from build123d import *

# Parameters (mm, degrees)
BOSS_EXTRUDE2_DEPTH      = 2
BOSS_EXTRUDE2_DEPTH_BACK = 2
SKETCH1_3_W              = 45
SKETCH1_3_H              = 20
BOSS_EXTRUDE3_DEPTH      = 35
M3_5_CLEARANCE_HOLE2_D   = 3.9
M6_CLEARANCE_HOLE2_D     = 6.6


with BuildPart() as part:
    # Sketch1<3> → Boss-Extrude2 (new, two sides: drawn at the far end of the back side and taken through both)
    with BuildSketch(Plane.XY.offset(-BOSS_EXTRUDE2_DEPTH_BACK)):
        with BuildLine():
            Line((-18.78, 17.478483309), (-8.78, 17.478483309))
            Line((-8.78, 17.478483309), (-8.78, 27.45))
            ThreePointArc((-8.78, 27.45), (-13.78, 32.45), (-18.78, 27.45))
            Line((-18.78, 27.45), (-18.78, 17.478483309))
        make_face()
        Polygon((-18.78, -10), (-18.78, -17.478483309), (-8.78, -17.478483309), (-8.78, 17.478483309), (-18.78, 17.478483309), (-18.78, 10), align=None)
        with BuildLine():
            Line((-8.78, -17.478483309), (-18.78, -17.478483309))
            Line((-18.78, -17.478483309), (-18.78, -27.45))
            ThreePointArc((-18.78, -27.45), (-13.78, -32.45), (-8.78, -27.45))
            Line((-8.78, -27.45), (-8.78, -17.478483309))
        make_face()
        with Locations((-41.28, 0)):
            Rectangle(SKETCH1_3_W, SKETCH1_3_H)
        Polygon((-63.78, -25), (-63.78, -10), (-63.78, 10), (-63.78, 25), (-66.78, 25), (-66.78, -25), align=None)
    extrude(amount=BOSS_EXTRUDE2_DEPTH + BOSS_EXTRUDE2_DEPTH_BACK)

    # Sketch1<4> → Boss-Extrude3 (add)
    with BuildSketch(Plane.XY):
        Polygon((-63.78, -25), (-63.78, -10), (-63.78, 10), (-63.78, 25), (-66.78, 25), (-66.78, -25), align=None)
    extrude(amount=BOSS_EXTRUDE3_DEPTH)

    # M3.5 Clearance Hole2 (through all)
    with Locations(Plane(origin=(0, 0, -2), x_dir=(-1, 0, 0), z_dir=(0, 0, -1))):
        with Locations((13.78, 27.45), (13.78, -27.45)):
            Hole(M3_5_CLEARANCE_HOLE2_D / 2)

    # M6 Clearance Hole2 (through all)
    with Locations(Plane(origin=(-63.78, 0, 0), x_dir=(0, 0, -1), z_dir=(1, 0, 0))):
        with Locations((-29, 19)):
            m6_clearance_hole2 = Hole(M6_CLEARANCE_HOLE2_D / 2)

    # Mirror1: M6 Clearance Hole2 across plane
    add(m6_clearance_hole2.mirror(Plane.ZX), mode=Mode.SUBTRACT)


solid = part.part
CAD build for the part. Positions are in the model's coordinates, mm. A direction names the side the tool comes from. Round coordinates to 2 decimals unless told otherwise and drop trailing zeros. Write each loop counter-clockwise with the first axis right and the second up, starting at its lowest first coordinate (ties: lowest second). Pieces come first, ordered by that corner, then holes.
(1) Mould opens along Y. For faces 5 (the face through (-65.3, 17.74, 32.05)), 6 (the face through (-13.67, 32.45, -0.03)), 7 (the face through (-8.78, 0, 0)) say: pulls with the +Y half, pulls with the -Y half, needs draft (parallel to the pull), parting line crosses it, or undercut.
(2) Slice it at C-C, the plane y = 0.5. Write the cut outline in (x, z).
(3) Slice it at A-A, the plane x = -13.78. Write the cut outline in (y, z), and give its area (3 significant figures).
(4) Probe line 1 along Y through (x, z) = (-65, 29); line 2 along X through (y, z) = (13, 29.5); line 3 along Y through (x, z) = (-13, -1). List the from-to ranges inside material, lowest first.
(5) Drop flat-ended pins along their axis: P1, Ø1.2, axis at x = -35, z = 1, coming from the +Y side; P2, Ø3, axis at y = -10.5, z = 9, coming from the +X side; P3, Ø2, axis at x = -48, z = 0.5, coming from the -Y side. Give the stop position or say it passes through.
(6) Slice it at D-D, the plane x = -32.5. Write the cut outline in (y, z).
(7) 3-axis set-ups, long thin cutter, end or side, ignore diameter. For faces 1 (the face through (-42, 10, 0)), 2 (the face through (-15.728, -27.364, 0.028)), 3 (the face through (-42, -10, 0)), 4 (the face through (-31, 0, 2)): which of +Z, -Z, +X, -X, +Y, -Y reach the whole face in a straight line?
(8) Slice it at B-B, the plane z = 29. Write the cut outline in (x, y), and give its area (3 significant figures).
From the geometry:
1. face 5: undercut
1. face 6: pulls with the +Y half
1. face 7: needs draft
2. outline: (-66.78, -2) - (-8.78, -2) - (-8.78, 2) - (-63.78, 2) - (-63.78, 35) - (-66.78, 35) - close
3. outline: (-32.45, -2) - (-29.4, -2) - (-29.4, 2) - (-32.45, 2) - close; (-25.5, -2) - (25.5, -2) - (25.5, 2) - (-25.5, 2) - close; (29.4, -2) - (32.45, -2) - (32.45, 2) - (29.4, 2) - close
3. area: 228 mm2
4. line 1: y = -25 to -22.3, -15.7 to 15.7, 22.3 to 25
4. line 2: x = -66.78 to -63.78
4. line 3: y = -32.39 to -29.24, -25.66 to 25.66, 29.24 to 32.39
5. P1: stops at y = 10
5. P2: stops at x = -63.78
5. P3: stops at y = -10
6. outline: (-10, -2) - (10, -2) - (10, 2) - (-10, 2) - close
7. face 1: +Z, -Z, +Y
7. face 2: +Z, -Z
7. face 3: +Z, -Z, -Y
7. face 4: +Z, +X, +Y, -Y
8. outline: (-66.78, -25) - (-63.78, -25) - (-63.78, -22.3) - (-66.78, -22.3) - close; (-66.78, -15.7) - (-63.78, -15.7) - (-63.78, 15.7) - (-66.78, 15.7) - close; (-66.78, 22.3) - (-63.78, 22.3) - (-63.78, 25) - (-66.78, 25) - close
8. area: 110 mm2
